```python
from build123d import *

# Parameters (mm, degrees)
F0_W     = 58.42
F0_H     = 5.715
F0_W_2   = 55.88
F0_H_2   = 3.175
F1_DEPTH = 6.35
F2_DEPTH = 5.334
F3_DEPTH = 1.016


with BuildPart() as f1:
    # F0 (on Top) → F1 (new body)
    with BuildSketch(Plane.XY):
        with BuildLine():
            Line((56.1975, 13.9065), (-0.3175, 13.9065))
            ThreePointArc((-0.3175, 13.9065), (-7.68131, 10.85631), (-10.7315, 3.4925))
            Line((-10.7315, 3.4925), (-10.7315, -0.3175))
            ThreePointArc((-10.7315, -0.3175), (-7.68131, -7.68131), (-0.3175, -10.7315))
            Line((-0.3175, -10.7315), (56.1975, -10.7315))
            ThreePointArc((56.1975, -10.7315), (63.56131, -7.68131), (66.6115, -0.3175))
            Line((66.6115, -0.3175), (66.6115, 3.4925))
            ThreePointArc((66.6115, 3.4925), (63.56131, 10.85631), (56.1975, 13.9065))
        make_face()
        with Locations((27.94, 1.5875)):
            Rectangle(F0_W, F0_H, mode=Mode.SUBTRACT)
        with Locations((27.94, 1.5875)):
            Rectangle(F0_W, F0_H)
        with Locations((27.94, 1.5875)):
            Rectangle(F0_W_2, F0_H_2, mode=Mode.SUBTRACT)
    extrude(amount=-F1_DEPTH)

    # F0 (on Top) → F2 (cut)
    with BuildSketch(Plane.XY):
        with BuildLine():
            Line((56.1975, 13.9065), (-0.3175, 13.9065))
            ThreePointArc((-0.3175, 13.9065), (-7.68131, 10.85631), (-10.7315, 3.4925))
            Line((-10.7315, 3.4925), (-10.7315, -0.3175))
            ThreePointArc((-10.7315, -0.3175), (-7.68131, -7.68131), (-0.3175, -10.7315))
            Line((-0.3175, -10.7315), (56.1975, -10.7315))
            ThreePointArc((56.1975, -10.7315), (63.56131, -7.68131), (66.6115, -0.3175))
            Line((66.6115, -0.3175), (66.6115, 3.4925))
            ThreePointArc((66.6115, 3.4925), (63.56131, 10.85631), (56.1975, 13.9065))
        make_face()
        with Locations((27.94, 1.5875)):
            Rectangle(F0_W, F0_H, mode=Mode.SUBTRACT)
    extrude(amount=-F2_DEPTH, mode=Mode.SUBTRACT)

    # F0 (on Top) → F3 (join)
    with BuildSketch(Plane.XY):
        with BuildLine():
            Line((56.1975, 13.9065), (-0.3175, 13.9065))
            ThreePointArc((-0.3175, 13.9065), (-7.68131, 10.85631), (-10.7315, 3.4925))
            Line((-10.7315, 3.4925), (-10.7315, -0.3175))
            ThreePointArc((-10.7315, -0.3175), (-7.68131, -7.68131), (-0.3175, -10.7315))
            Line((-0.3175, -10.7315), (56.1975, -10.7315))
            ThreePointArc((56.1975, -10.7315), (63.56131, -7.68131), (66.6115, -0.3175))
            Line((66.6115, -0.3175), (66.6115, 3.4925))
            ThreePointArc((66.6115, 3.4925), (63.56131, 10.85631), (56.1975, 13.9065))
        make_face()
        with Locations((27.94, 1.5875)):
            Rectangle(F0_W, F0_H, mode=Mode.SUBTRACT)
    extrude(amount=-F3_DEPTH)


solid = f1.part
```
Part model, mm, in its own coordinate system. A direction names the side the tool comes from. Round coordinates to 2 decimals unless told otherwise and drop trailing zeros. Write each loop counter-clockwise with the first axis right and the second up, starting at its lowest first coordinate (ties: lowest second). Pieces come first, ordered by that corner, then holes. Notation, with made-up numbers: (19.25, -8) -> (39.25, -8) arc R20 cw to (39.25, -3) -> close; hole circle Ø11 at (6.5, 74.5). An arc over 180 degrees is marked (long way). Return JSON: item names as keys, results as strings. Group by question number.
Q1. Pin check, flat tips, straight feed: pin 1 (1.3 mm diameter, centred on x = 30.5, z = -2.5, fed in from -Y); pin 2 (1.3 mm diameter, centred on x = 16, z = -4, fed in from +Y) (3 decimals). Stop position of each tip, or through.
Q2. Mould opens along Z. For faces 5 (the flat face through (28, -1.27, -3)), 6 (the flat face through (27, 4, 0)), 7 (the cylindrical face through (63.642, 10.775, -0.501)) say: pulls with the +Z half, pulls with the -Z half, needs draft (parallel to the pull), parting line crosses it, or undercut.
Q3. Which spindle directions (+Z, -Z, +X, -X, +Y, -Y) get a long thin tool onto all of the face, cutting with end or side? Do faces 1 (the flat face through (0, 2, -3)), 2 (the flat face through (-1.27, 2, -3)), 3 (the flat face through (28, 4.445, -3)), 4 (the flat face through (57.15, 2, -3)). Say none if no direction does.
Q4. Saw through at C-C on z = -2.5. Write the cut outline in (x, y) (3 decimals), plus the area to 3 significant figures.
Q5. Saw through at A-A on y = 2.25. Write the cut outline in (x, z), plus the area to 3 significant figures.
Q6. Probe L1, parallel to Y at x = 53, z = -4 (3 decimals); L2, parallel to Z at x = 37.5, y = 5.75; L3, parallel to X at y = 1.75, z = -0.75. List the from-to ranges inside material, lowest first. Write a range as [from, to].
Q7. Saw through at D-D on y = -4.25. Write the cut outline in (x, z).
Answer:
{
 "1": {"pin 1": "y = -1.27", "pin 2": "y = 4.445"},
 "2": {"face 5": "undercut", "face 6": "pulls with the +Z half", "face 7": "needs draft"},
 "3": {"face 1": "+Z, -Z", "face 2": "-X, +Y, -Y", "face 3": "+X, -X, +Y", "face 4": "+X, +Y, -Y"},
 "4": {"outline": "(-1.27, -1.27) -> (57.15, -1.27) -> (57.15, 4.445) -> (-1.27, 4.445) -> close; hole (0, 0) -> (55.88, 0) -> (55.88, 3.175) -> (0, 3.175) -> close", "area": "156 mm2"},
 "5": {"outline": "(-10.73, -6.35) -> (0, -6.35) -> (0, 0) -> (-10.73, 0) -> (-10.73, -1.02) -> (-1.27, -1.02) -> (-1.27, -5.33) -> (-10.73, -5.33) -> close; (55.88, -6.35) -> (66.61, -6.35) -> (66.61, -5.33) -> (57.15, -5.33) -> (57.15, -1.02) -> (66.61, -1.02) -> (66.61, 0) -> (55.88, 0) -> close", "area": "54.6 mm2"},
 "6": {"L1": "[-1.27, 0], [3.175, 4.445]", "L2": "[-6.35, -5.33], [-1.02, 0]", "L3": "[-10.73, 0], [55.88, 66.61]"},
 "7": {"outline": "(-9.96, -6.35) -> (65.84, -6.35) -> (65.84, -5.33) -> (-9.96, -5.33) -> close; (-9.96, -1.02) -> (65.84, -1.02) -> (65.84, 0) -> (-9.96, 0) -> close"}
}
